```python
from build123d import *

# Parameters (mm, degrees)
F1_DEPTH = 16.933333
F2_W     = 49.271976
F2_H     = 22.225
F3_DEPTH = 3.175
F4_W     = 49.271976
F4_H     = 22.225
F5_DEPTH = 3.175


with BuildPart() as f1:
    # F0 (on Right) → F1 (new body)
    with BuildSketch(Plane.YZ):
        Polygon((21.467701, 5.752253), (0, 0), (-21.887352, 3.859331), (-21.887352, -3.175847), (27.384624, -3.175847), (27.384624, 15.277253), (21.467701, 15.277253), align=None)
    extrude(amount=F1_DEPTH)

    # F2 (on Right) → F3 (join)
    with BuildSketch(Plane.YZ):
        with Locations((2.748636, 7.936653)):
            Rectangle(F2_W, F2_H)
    extrude(amount=-F3_DEPTH)

    # F4 (on face) → F5 (join)
    with BuildSketch(Plane.YZ.offset(16.933333)):
        with Locations((2.748636, 7.936653)):
            Rectangle(F4_W, F4_H)
    extrude(amount=F5_DEPTH)


solid = f1.part
```
Can you work these out from the model? Positions are in its coordinate system, mm. A direction names the side the tool comes from. Round coordinates to 2 decimals unless told otherwise and drop trailing zeros. Loops run counter-clockwise (first coordinate to the right, second up) from the corner with the lowest first, then second, coordinate; pieces in that order, holes last. Notation, with made-up numbers: (-35.75, -11) -> (5.25, -11) arc R23 cw to (5.25, 8) -> close; hole circle Ø2 at (39.25, 23.25). An arc over 180 degrees is marked (long way). One line per item, written item: value. Start each with the question number.
1. For pin 1 (1.8 mm diameter, centred on x = 10.5, y = 24.5, fed in from +Z); pin 2 (1.5 mm diameter, centred on x = 6, y = 15.5, fed in from +Z), each with a flat end and sliding along its axis, tell me the tip position at first contact or that it passes through.
2. If we section it at D-D, the plane x = 10.75: Write out the boundary of the cut face in (y, z), then the cut area to 3 significant figures.
3. If we mould it in two halves opening along Y, with no side actions, what happens to faces 5 (the flat face through (8.348, -10.79, 1.903)), 6 (the flat face through (-3.175, 2, 8)), 7 (the flat face through (8, 27.385, 8))? For each: pulls with the +Y half, pulls with the -Y half, needs draft (parallel to the pull), parting line crosses it, or undercut.
4. For faces 1 (the flat face through (8.348, 10.884, 2.916)), 2 (the flat face through (8, 24, 15.277)), 3 (the flat face through (18, 2, 19.049)), 4 (the flat face through (8, 21.468, 11)), which set-ups out of +Z, -Z, +X, -X, +Y, -Y let a thin tool reach every point of the face, with its end or its side?
5. If we section it at C-C, the plane y = -4.5: Write out the boundary of the cut face in (x, z) (3 decimals), then the cut area to 3 significant figures.
6. If I drill on probe 1 along X at (y, z) = (19, 13) (3 decimals); probe 2 along Y at (x, z) = (9.25, 9.75); probe 3 along Z at (x, y) = (1.75, 21.5), over which ranges is the centre line in solid material (lowest first)?
7. If we section it at A-A, the plane z = 16.5: Write out the boundary of the cut face in (x, y) (3 decimals), then the cut area to 3 significant figures.
8. If we section it at B-B, the plane z = 7.75: Write out the boundary of the cut face in (x, y) (3 decimals), then the cut area to 3 significant figures.
Calculated:
1. pin 1: stops at z = 15.28
1. pin 2: stops at z = 4.35
2. outline: (-21.89, -3.18) -> (27.38, -3.18) -> (27.38, 15.28) -> (21.47, 15.28) -> (21.47, 5.75) -> (0, 0) -> (-21.89, 3.86) -> close
2. area: 351 mm²
3. face 5: undercut
3. face 6: needs draft
3. face 7: pulls with the +Y half
4. face 1: +Z
4. face 2: +Z, +Y, -Y
4. face 3: +Z, +X, -X, +Y, -Y
4. face 4: +Z, -Y
5. outline: (-3.175, -3.176) -> (20.108, -3.176) -> (20.108, 19.049) -> (16.933, 19.049) -> (16.933, 0.793) -> (0, 0.793) -> (0, 19.049) -> (-3.175, 19.049) -> close
5. area: 208 mm²
6. probe 1: x = -3.175 to 0, 16.933 to 20.108
6. probe 2: y = 21.47 to 27.38
6. probe 3: z = -3.18 to 15.28
7. outline: (-3.175, -21.887) -> (0, -21.887) -> (0, 27.385) -> (-3.175, 27.385) -> close; (16.933, -21.887) -> (20.108, -21.887) -> (20.108, 27.385) -> (16.933, 27.385) -> close
7. area: 313 mm²
8. outline: (-3.175, -21.887) -> (0, -21.887) -> (0, 21.468) -> (16.933, 21.468) -> (16.933, -21.887) -> (20.108, -21.887) -> (20.108, 27.385) -> (-3.175, 27.385) -> close
8. area: 413 mm²
